Work out the finished part from the listing and answer in its coordinate system (mm). Face numbers are marked on the shaded views. A direction names the side the tool comes from. Coordinates: 2 decimals unless noted, no trailing zeros. Loops run counter-clockwise (first coordinate to the right, second up) from the corner with the lowest first, then second, coordinate; pieces in that order, holes last. Notation, with made-up numbers: (87.25, 17.25) - (130.25, 17.25) arc R12 ccw to (130.25, 33.25) - close; hole circle Ø6 at (-11, -33). An arc over 180 degrees is marked (long way). Write each question's results on one line, items separated by ' | '. Start each with the question number.
Item 1: Section A-A, the plane z = 7 is taken. Write down the section's boundary in (x, y).
Item 2: Each of these flat-tipped pins is pushed along its axis until it touches: pin 1 Ø9 at (y, z) = (-15, 40) entering from +X; pin 2 Ø1.5 at (x, z) = (37, 42) entering from +Y; pin 3 Ø10 at (x, z) = (47.5, 25.5) entering from +Y; pin 4 Ø3 at (y, z) = (46, 37) entering from -X. Where does it stop, or does it pass through?
Item 3: Section B-B, the plane y = 6 is taken. Write down the section's boundary in (x, z), plus the area to 3 significant figures.
Item 4: A tool of negligible diameter and unlimited length cuts with its end or side. For the marked faces 1 and 2, from which of +Z, -Z, +X, -X, +Y, -Y can it reach the whole face along a straight path? Write none if from no direction.
Item 5: For a pull along Y with two mould halves and no side action, classify the marked faces 3, 4 and 5 as +Y half, -Y half, draft (parallel to the pull), parting line (faces both ways), or undercut.
Item 6: Section C-C, the plane y = 62 is taken. Count the separate pieces of the cut face and the enclosed holes in it, plus the area to 3 significant figures.
Item 7: Consider probe 1 along Z at (x, y) = (2.9, -15); probe 2 along X at (y, z) = (-12, 32.5); probe 3 along Y at (x, z) = (16, 21). Determine where each line is inside the solid, lowest interval first. Write a range as [from, to].
from build123d import *

# Parameters (mm, degrees)
BOSS_EXTRUDE1_DEPTH     = 50
SKETCH2_R               = 15
CUT_EXTRUDE1_DEPTH      = 60
CHAMFER1_SIZE           = 5
CUT_EXTRUDE2_DEPTH      = 128.713132763
CUT_EXTRUDE2_DEPTH_BACK = 128.713132763
SKETCH3_R               = 5
FILLET2_R               = 10
FILLET3_R               = 25


with BuildPart() as part:
    # Sketch1 → Boss-Extrude1 (new body)
    with BuildSketch(Plane.XY):
        with BuildLine():
            Line((5, -25), (5, 0))
            Line((5, 0), (35, 0))
            Line((35, 0), (35, -25))
            Line((35, -25), (40, -25))
            Line((40, -25), (40, 0))
            Line((40, 0), (40, 12.914909334))
            Line((40, 12.914909334), (85.43033171, 44.72557006))
            Line((85.43033171, 44.72557006), (56.751509892, 85.683172275))
            Line((56.751509892, 85.683172275), (40.368469006, 74.211643548))
            Line((40.368469006, 74.211643548), (54.707879915, 53.732842441))
            ThreePointArc((54.707879915, 53.732842441), (53.480001875, 46.769200037), (46.516359472, 47.997078077))
            Line((46.516359472, 47.997078077), (32.176948563, 68.475879184))
            Line((32.176948563, 68.475879184), (0, 45.945337244))
            Line((0, 45.945337244), (0, 0))
            Line((0, 0), (0, -25))
            Line((0, -25), (5, -25))
        make_face()
    extrude(amount=BOSS_EXTRUDE1_DEPTH)

    # Sketch2 → Cut-Extrude1 (cut)
    with BuildSketch(Plane(origin=(78.338757076, 54.853388238, 0), x_dir=(0, 0, -1), z_dir=(0.8191520442889928, 0.5735764363510449, 0))):
        with Locations(Location((-25, 12.636216929, 0), (0, 0, 90))):
            Circle(SKETCH2_R)
    extrude(amount=-CUT_EXTRUDE1_DEPTH, mode=Mode.SUBTRACT)

    # Chamfer1
    chamfer1_edges = [part.edges().sort_by_distance(p)[0] for p in [
        (30.545444689, 18.502504322, 25),
    ]]
    chamfer(chamfer1_edges, length=CHAMFER1_SIZE)

    # Sketch3 → Cut-Extrude2 (cut, two sides: drawn at the far end of the back side and taken through both)
    with BuildSketch(Plane(origin=(5, 0, 0), x_dir=(0, 0, -1), z_dir=(1, 0, 0)).offset(-CUT_EXTRUDE2_DEPTH_BACK)):
        with Locations((-40, -15)):
            Circle(SKETCH3_R)
        with Locations((-10, -15)):
            Circle(SKETCH3_R)
    extrude(amount=CUT_EXTRUDE2_DEPTH + CUT_EXTRUDE2_DEPTH_BACK, mode=Mode.SUBTRACT)

    # Fillet2
    fillet2_edges = [part.edges().sort_by_distance(p)[0] for p in [
        (37.5, -25, 0),
        (2.5, -25, 0),
        (2.5, -25, 50),
        (37.5, -25, 50),
    ]]
    fillet(fillet2_edges, radius=FILLET2_R)

    # Fillet3
    # the kernel refuses this fillet: 25 mm, written as the material it takes off along each edge
    with BuildSketch(Plane(origin=(83.373951331, 104.324406456, 0), x_dir=(0.5735764363510446, -0.8191520442889929, 0), z_dir=(-0.8191520442889929, -0.5735764363510447, 0)), Plane(origin=(83.373951331, 104.324406456, 50), x_dir=(0, 0, -1), z_dir=(-0.8191520442889929, -0.5735764363510447, 0))) as fillet3_piece_1:
        with BuildLine():
            CenterArc((FILLET3_R, FILLET3_R), FILLET3_R, 180, 90)
            Line((0, FILLET3_R), (0, 0))
            Line((0, 0), (FILLET3_R, 0))
        make_face()
    extrude(amount=164.28080115, mode=Mode.SUBTRACT)
    with BuildSketch(Plane(origin=(107.94851266, 121.531699547, 0), x_dir=(0.573576436351046, -0.8191520442889918, 0), z_dir=(-0.8191520442889919, -0.5735764363510462, 0)), Plane(origin=(107.94851266, 121.531699547, 50), x_dir=(0, 0, -1), z_dir=(-0.8191520442889919, -0.5735764363510462, 0))) as fillet3_piece_2:
        with BuildLine():
            CenterArc((FILLET3_R, FILLET3_R), FILLET3_R, 180, 90)
            Line((0, FILLET3_R), (0, 0))
            Line((0, 0), (FILLET3_R, 0))
        make_face()
    extrude(amount=145, mode=Mode.SUBTRACT)
    with BuildSketch(Plane(origin=(-11.197002768, -22.933617938, 0), x_dir=(-0.5735764363510454, 0.8191520442889921, 0), z_dir=(0.8191520442889924, 0.5735764363510455, 0))) as fillet3_piece_3_section:
        with BuildLine():
            CenterArc((FILLET3_R, FILLET3_R), FILLET3_R, 180, 90)
            Line((0, FILLET3_R), (0, 0))
            Line((0, 0), (FILLET3_R, 0))
        make_face()
    fillet3_piece_3 = extrude(amount=180.46019451, mode=Mode.PRIVATE)
    fillet3_piece_3 = split(fillet3_piece_3, bisect_by=Plane(origin=(40, 25.184030637, 6.00422592), z_dir=(1, 0, 0)), keep=Keep.TOP, mode=Mode.PRIVATE)
    add(fillet3_piece_3, mode=Mode.SUBTRACT)
    with BuildSketch(Plane(origin=(-11.197002768, -22.933617938, 50), x_dir=(0, 0, -1), z_dir=(0.8191520442889924, 0.5735764363510455, 0))) as fillet3_piece_4_section:
        with BuildLine():
            CenterArc((FILLET3_R, FILLET3_R), FILLET3_R, 180, 90)
            Line((0, FILLET3_R), (0, 0))
            Line((0, 0), (FILLET3_R, 0))
        make_face()
    fillet3_piece_4 = extrude(amount=180.46019451, mode=Mode.PRIVATE)
    fillet3_piece_4 = split(fillet3_piece_4, bisect_by=Plane(origin=(40, 25.184030637, 43.99577408), z_dir=(1, 0, 0)), keep=Keep.TOP, mode=Mode.PRIVATE)
    add(fillet3_piece_4, mode=Mode.SUBTRACT)


solid = part.part
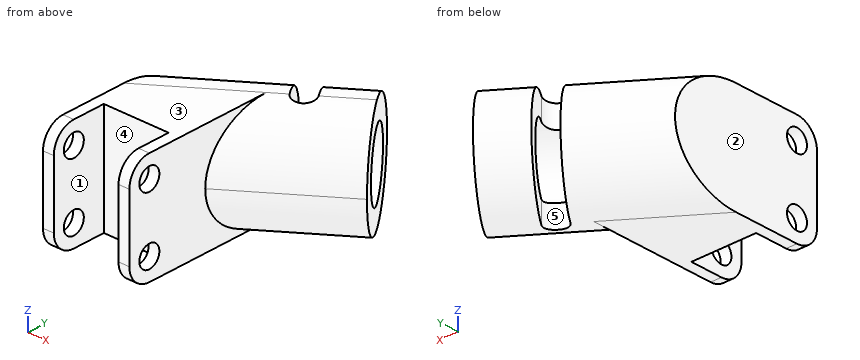
Answer key:
1) outline: (0, -24.54) - (5, -24.54) - (5, -19) - (0, -19) - close; (0, -11) - (5, -11) - (5, 0) - (35, 0) - (35, -11) - (40, -11) - (40, 22.25) - (81.04, 50.99) - (61.14, 79.42) - (44.76, 67.94) - (54.71, 53.73) arc R5 cw to (46.52, 48) - (36.57, 62.21) - (0, 36.61) - close; (35, -24.54) - (40, -24.54) - (40, -19) - (35, -19) - close
2) pin 1: passes through | pin 2: stops at y = 62.66 | pin 3: stops at y = 82.7 | pin 4: stops at x = 2.88
3) outline: (0, 0) - (40, 0) - (40, 50) - (0, 50) - close | area: 2,000 mm^2
4) face 1: +Z, -Z, -Y | face 2: +Z, -Z, -X, +Y, -Y
5) face 3: draft | face 4: -Y half | face 5: undercut
6) separate pieces: 3 | enclosed holes: 0 | area: 855 mm^2
7) probe 1: z = [0, 5], [15, 35], [45, 50] | probe 2: x = [0, 5], [35, 40] | probe 3: y = [0, 56.76]
